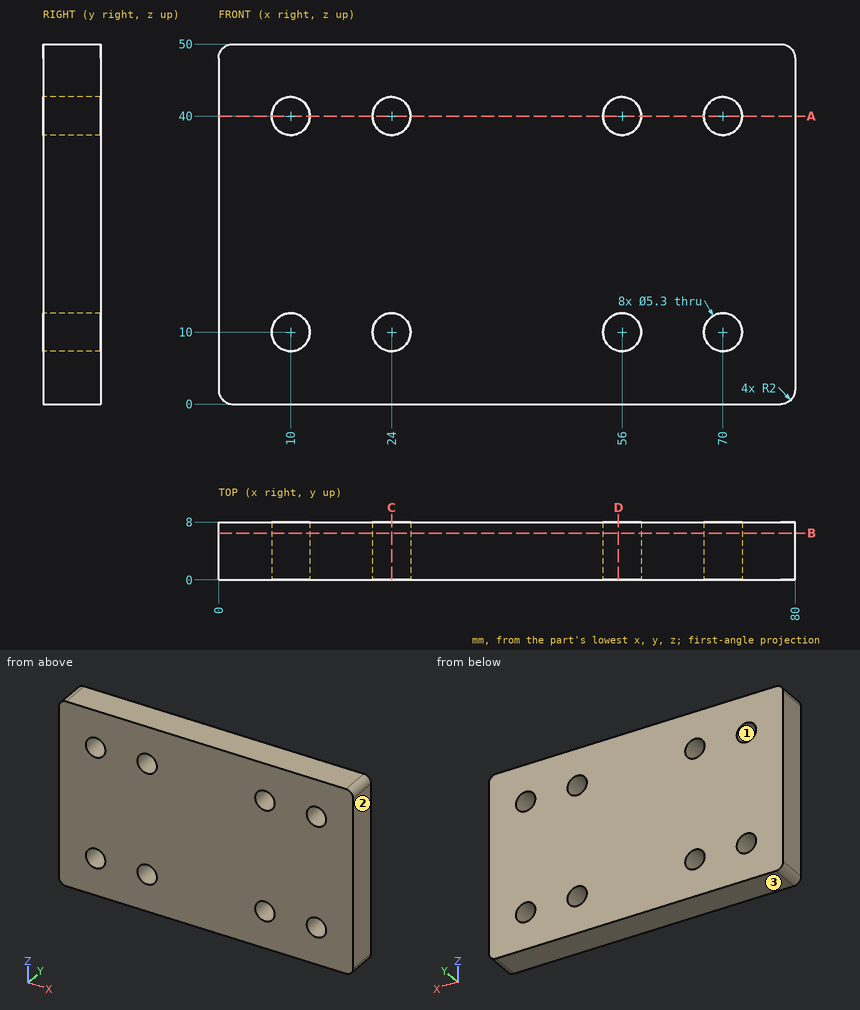
The drawing under review shows one solid part. Ordinate dimensions are in mm from its lowest x, y, z. Coordinates: 2 decimals unless noted, no trailing zeros. Loops run counter-clockwise (first coordinate to the right, second up) from the corner with the lowest first, then second, coordinate; pieces in that order, holes last. Notation, with made-up numbers: (48.5, 26.25) - (65.5, 26.25) arc R18 cw to (65.5, 33.25) - close; hole circle Ø4 at (44.25, 43.25). An arc over 180 degrees is marked (long way). Use CSV: the item, a comma, the result in double quotes. Start each with the question number.
1. Mouldability with a two-part tool opening along Z and no side actions: class the marked faces 1, 2 and 3 as released by +Z, released by -Z, zero draft, split by the parting line, or undercut.
2. Add section D-D on x = 55.5. Give the boundary of the cut face in (y, z).
3. Add section A-A on z = 40. Give the boundary of the cut face in (x, y), plus the area to 3 significant figures.
4. Add section B-B on y = 6.5. Count the separate pieces of the cut face and the enclosed holes in it, plus the area to 3 significant figures.
5. To check wall thickness, follow probe 1 along Z at (x, y) = (70, 4.25); probe 2 along X at (y, z) = (6.25, 10); probe 3 along X at (y, z) = (5, 12). State the ranges of each line that lie inside material, in increasing order.
6. Add section C-C on x = 24. Give the boundary of the cut face in (y, z), plus the area to 3 significant figures.
Resolved:
1,face 1,"undercut"
1,face 2,"zero draft"
1,face 3,"released by -Z"
2,outline,"(0, 0) - (8, 0) - (8, 7.4) - (0, 7.4) - close; (0, 12.6) - (8, 12.6) - (8, 37.4) - (0, 37.4) - close; (0, 42.6) - (8, 42.6) - (8, 50) - (0, 50) - close"
3,outline,"(0, 0) - (7.35, 0) - (7.35, 8) - (0, 8) - close; (12.65, 0) - (21.35, 0) - (21.35, 8) - (12.65, 8) - close; (26.65, 0) - (53.35, 0) - (53.35, 8) - (26.65, 8) - close; (58.65, 0) - (67.35, 0) - (67.35, 8) - (58.65, 8) - close; (72.65, 0) - (80, 0) - (80, 8) - (72.65, 8) - close"
3,area,"470 mm2"
4,separate pieces,"1"
4,enclosed holes,"8"
4,area,"3,820 mm2"
5,probe 1,"0 to 7.35, 12.65 to 37.35, 42.65 to 50"
5,probe 2,"0 to 7.35, 12.65 to 21.35, 26.65 to 53.35, 58.65 to 67.35, 72.65 to 80"
5,probe 3,"0 to 8.26, 11.74 to 22.26, 25.74 to 54.26, 57.74 to 68.26, 71.74 to 80"
6,outline,"(0, 0) - (8, 0) - (8, 7.35) - (0, 7.35) - close; (0, 12.65) - (8, 12.65) - (8, 37.35) - (0, 37.35) - close; (0, 42.65) - (8, 42.65) - (8, 50) - (0, 50) - close"
6,area,"315 mm2"
